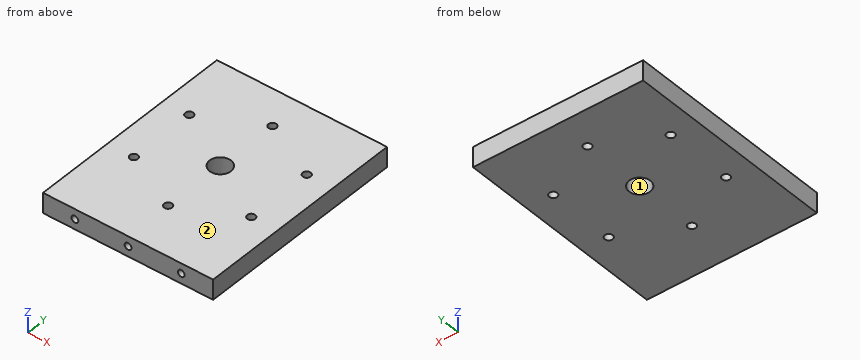
```python
from build123d import *

# Parameters (mm, degrees)
SKETCH1_W                  = 101.6
SKETCH1_H                  = 127
SKETCH1_R                  = 6.35
BOSS_EXTRUDE1_DEPTH        = 12.0000014
SKETCH2_R                  = 2.38125
CUT_EXTRUDE1_DEPTH         = 138.308557758
SKETCH3_R                  = 1.27
CUT_EXTRUDE2_DEPTH         = 12.7
F_10_32_TAPPED_HOLE3_D     = 4.0386
F_10_32_TAPPED_HOLE3_DEPTH = 12.7
F_10_32_TAPPED_HOLE3_TIP   = 1.213317848


with BuildPart() as part:
    # Sketch1 → Boss-Extrude1 (new body)
    with BuildSketch(Plane.XY):
        with Locations((0, 63.5)):
            Rectangle(SKETCH1_W, SKETCH1_H)
        with Locations((0, 67.3749986)):
            Circle(SKETCH1_R, mode=Mode.SUBTRACT)
    extrude(amount=BOSS_EXTRUDE1_DEPTH)

    # Sketch2 → Cut-Extrude1 (cut, through all)
    with BuildSketch(Plane(origin=(0, 0, 0), x_dir=(-1, 0, 0), z_dir=(0, 0, -1))):
        with Locations((0, 105.4749986)):
            Circle(SKETCH2_R)
        with Locations((0, 29.2749986)):
            Circle(SKETCH2_R)
        with Locations((-35.057790877, 87.6156236)):
            Circle(SKETCH2_R)
        with Locations((-35.057790877, 47.1343736)):
            Circle(SKETCH2_R)
        with Locations((35.057790877, 47.1343736)):
            Circle(SKETCH2_R)
        with Locations((35.057790877, 87.6156236)):
            Circle(SKETCH2_R)
    extrude(amount=-CUT_EXTRUDE1_DEPTH, mode=Mode.SUBTRACT)

    # Sketch3 → Cut-Extrude2 (cut)
    with BuildSketch(Plane.XZ):
        with Locations(Location((31.75, 6.0000007, 0), (0, 0, 270))):
            Circle(SKETCH3_R)
        with Locations(Location((0, 6.0000007, 0), (0, 0, 270))):
            Circle(SKETCH3_R)
        with Locations(Location((-31.75, 6.0000007, 0), (0, 0, 270))):
            Circle(SKETCH3_R)
    extrude(amount=-CUT_EXTRUDE2_DEPTH, mode=Mode.SUBTRACT)

    # #10-32 Tapped Hole3
    with Locations(Plane(origin=(0, 0, 0), x_dir=(-1, 0, 0), z_dir=(0, -1, 0))):
        with Locations((-31.75, -6.0000007), (0, -6.0000007), (31.75, -6.0000007)):
            Hole(F_10_32_TAPPED_HOLE3_D / 2, depth=F_10_32_TAPPED_HOLE3_DEPTH)
            with Locations((0, 0, -(F_10_32_TAPPED_HOLE3_DEPTH + F_10_32_TAPPED_HOLE3_TIP / 2))):  # 118° drill point
                Cone(0, F_10_32_TAPPED_HOLE3_D / 2, F_10_32_TAPPED_HOLE3_TIP, mode=Mode.SUBTRACT)


solid = part.part
```
Work out the finished part from the listing and answer in its coordinate system (mm). Face numbers are marked on the shaded views. Give positions to 0.01 mm unless a question says otherwise; leave off trailing zeros. Write each loop counter-clockwise with the first axis right and the second up, starting at its lowest first coordinate (ties: lowest second). Pieces come first, ordered by that corner, then holes. Notation, with made-up numbers: (-20.5, -12) -> (-7.5, -12) arc R23 cw to (-7.5, 22) -> close; hole circle Ø1 at (8.5, 14.5). An arc over 180 degrees is marked (long way). Write each question's results on one line, items separated by ' | '.
1. Find section A-A on y = 66. Determine the outline of the cut face in (x, z).
Data:
outline: (-50.8, 0) -> (-6.2, 0) -> (-6.2, 12) -> (-50.8, 12) -> close; (6.2, 0) -> (50.8, 0) -> (50.8, 12) -> (6.2, 12) -> close
2. Determine the mould class of the marked faces 1 and 2 for opening direction X: +X half, -X half, draft (parallel to the pull), parting line (faces both ways), or undercut.
Data:
face 1: undercut | face 2: draft
3. Find section B-B on x = -5. Determine the outline of the cut face in (y, z).
Data:
outline: (0, 0) -> (63.46, 0) -> (63.46, 12) -> (0, 12) -> close; (71.29, 0) -> (127, 0) -> (127, 12) -> (71.29, 12) -> close
4. Straight lines are drawn through the part: L1, parallel to Y at x = 0, z = 8.75 (3 decimals); L2, parallel to Y at x = -0.5, z = 4.75; L3, parallel to Z at x = 31, y = 10.5. For each, find the intervals that lie inside material, in ascending order.
Data:
L1: 0 to 26.894, 31.656 to 61.025, 73.725 to 103.094, 107.856 to 127 | L2: 13.1 to 26.95, 31.6 to 61.04, 73.71 to 103.15, 107.8 to 127 | L3: 0 to 4.13, 7.87 to 12
5. Find section C-C on z = 6. Give the number of separate pieces and of enclosed holes in the cut face, and give its area (3 significant figures).
Data:
separate pieces: 1 | enclosed holes: 7 | area: 12,500 mm^2
